```python
from build123d import *

# Parameters (mm, degrees)
SKETCH_1_W      = 5
SKETCH_1_H      = 2.75
EXTRUDE_1_DEPTH = 2.75


with BuildPart() as part:
    # 草图1 → 凸台-拉伸1 (new body)
    with BuildSketch(Plane.XY):
        Polygon((95, 100), (100, 100), (100, 102.75), (95, 102.75), (95, 102.449578136), align=None)
        Polygon((3, 3), (3, 0), (97, 0), (97, 3), (100, 3), (100, 100), (95, 100), (5, 100), (0, 100), (0, 3), align=None)
        with Locations((2.5, 101.375)):
            Rectangle(SKETCH_1_W, SKETCH_1_H)
        Polygon((0, 0), (0, -30), (10, -30), (30, -30), (30, -27), (50, -27), (70, -27), (70, -30), (90, -30), (100, -30), (100, 0), (97, 0), (3, 0), align=None)
        Polygon((30, -30), (10, -30), (10, -33), (90, -33), (90, -30), (70, -30), (50, -30), align=None)
    extrude(amount=EXTRUDE_1_DEPTH)


solid = part.part
```
Could you check a few things on this model? Use its own coordinates, in mm. A direction names the side the tool comes from. Coordinates: 2 decimals unless noted, no trailing zeros. Write each loop counter-clockwise with the first axis right and the second up, starting at its lowest first coordinate (ties: lowest second). Pieces come first, ordered by that corner, then holes. Notation, with made-up numbers: (45.5, -39) -> (104.5, -39) arc R5 cw to (104.5, -33) -> close; hole circle Ø5 at (37, 33). An arc over 180 degrees is marked (long way). Return JSON: item names as keys, results as strings.
(1) Imagine slicing it at D-D, the plane x = 17.5. Please give me the cut outline in (y, z), then the cut area to 3 significant figures.
Numbers:
{"outline": "(-33, 0) -> (100, 0) -> (100, 2.75) -> (-33, 2.75) -> close", "area": "366 mm2"}
(2) I need wall thicknesses on L1, parallel to Y at x = 46, z = 1; L2, parallel to Y at x = 13.5, z = 0.35; L3, parallel to Y at x = 8.5, z = 2.55. Which ranges of each line are inside material? Lowest first, please.
Numbers:
{"L1": "y = -33 to -30, -27 to 100", "L2": "y = -33 to 100", "L3": "y = -30 to 100"}
(3) Imagine slicing it at C-C, the plane x = 7.5. Please give me the cut outline in (y, z), then the cut area to 4 significant figures.
Numbers:
{"outline": "(-30, 0) -> (100, 0) -> (100, 2.75) -> (-30, 2.75) -> close", "area": "357.5 mm2"}
(4) Imagine slicing it at A-A, the plane z = 2. Please give me the cut outline in (x, y), then the cut area to 3 significant figures.
Numbers:
{"outline": "(0, -30) -> (10, -30) -> (10, -33) -> (90, -33) -> (90, -30) -> (100, -30) -> (100, 0) -> (97, 0) -> (97, 3) -> (100, 3) -> (100, 102.75) -> (95, 102.75) -> (95, 100) -> (5, 100) -> (5, 102.75) -> (0, 102.75) -> (0, 3) -> (3, 3) -> (3, 0) -> (0, 0) -> close; hole (30, -30) -> (70, -30) -> (70, -27) -> (30, -27) -> close", "area": "13,100 mm2"}
(5) Which directions (+Z, -Z, +X, -X, +Y, -Y) give clear straight access to the entire face, cutting with the end or side of a thin tool? Please do faces 4 (the flat face through (51, 100, 1)), 5 (the flat face through (5, -30, 1)), 6 (the flat face through (3, 2, 1)).
Numbers:
{"face 4": "+Z, -Z, +Y", "face 5": "+Z, -Z, -X, -Y", "face 6": "+Z, -Z, -X"}
(6) Imagine slicing it at B-B, the plane x = 64.5. Please give me the cut outline in (y, z).
Numbers:
{"outline": "(-33, 0) -> (-30, 0) -> (-30, 2.75) -> (-33, 2.75) -> close; (-27, 0) -> (100, 0) -> (100, 2.75) -> (-27, 2.75) -> close"}
(7) I'm going to push flat-ended pins straight in: pin 1 (1.4 mm diameter, centred on x = 2.5, z = 1.5, fed in from -Y); pin 2 (0.8 mm diameter, centred on x = 57.5, z = 2, fed in from +Y); pin 3 (1.4 mm diameter, centred on y = -31.5, z = 2, fed in from +X). Where does each tip first touch, or does it pass through?
Numbers:
{"pin 1": "stops at y = -30", "pin 2": "stops at y = 100", "pin 3": "stops at x = 90"}
(8) We'd pull the mould along Y, two halves only. Please class faces 1 (the flat face through (2, 102.75, 1)), 2 (the flat face through (95, 101, 1)), 3 (the flat face through (99, 0, 1)): +Y half, -Y half, draft (parallel to the pull), parting line (faces both ways), or undercut.
Numbers:
{"face 1": "+Y half", "face 2": "draft", "face 3": "undercut"}
